from build123d import *

# Parameters (mm, degrees)
BOSS_EXTRUDE1_DEPTH     = 22.5
SKETCH2_R               = 7
CUT_EXTRUDE1_DEPTH      = 142.089510595
CUT_EXTRUDE2_DEPTH      = 150.198693024
CUT_EXTRUDE2_DEPTH_BACK = 150.198693024
SKETCH5_R               = 7
CHAMFER2_SIZE           = 1
FILLET2_R               = 1.5


with BuildPart() as part:
    # Sketch1 → Boss-Extrude1 (new, symmetric)
    with BuildSketch(Plane.XY):
        with BuildLine():
            Line((-74, -9), (-74, 9))
            Line((-74, 9), (-45, 9))
            Line((-45, 9), (-45, 127))
            Line((-45, 127), (-1, 127))
            Line((-1, 127), (-1, 100.983328701))
            ThreePointArc((-1, 100.983328701), (0, 41), (1, 100.983328701))
            Line((1, 100.983328701), (1, 127))
            Line((1, 127), (45, 127))
            Line((45, 127), (45, 9))
            Line((45, 9), (74, 9))
            Line((74, 9), (74, -9))
            Line((74, -9), (-74, -9))
        make_face()
    extrude(amount=BOSS_EXTRUDE1_DEPTH, both=True)

    # Sketch2 → Cut-Extrude1 (cut, through all)
    with BuildSketch(Plane(origin=(0, 9, 0), x_dir=(1, 0, 0), z_dir=(0, 1, 0))):
        with Locations(Location((60, 0, 0), (0, 0, 180))):
            Circle(SKETCH2_R)
        with Locations((-60, 0)):
            Circle(SKETCH2_R)
    extrude(amount=-CUT_EXTRUDE1_DEPTH, mode=Mode.SUBTRACT)

    # Sketch5 → Cut-Extrude2 (cut, two sides: drawn at the far end of the back side and taken through both)
    with BuildSketch(Plane(origin=(-1, 0, 0), x_dir=(0, 0, -1), z_dir=(1, 0, 0)).offset(-CUT_EXTRUDE2_DEPTH_BACK)):
        with Locations(Location((0.330734984, 113.991664351, 0), (0, 0, 90))):
            Circle(SKETCH5_R)
    extrude(amount=CUT_EXTRUDE2_DEPTH + CUT_EXTRUDE2_DEPTH_BACK, mode=Mode.SUBTRACT)

    # Chamfer2
    chamfer2_edges = [part.edges().sort_by_distance(p)[0] for p in [
        (0, 41, -22.5),
        (0, 41, 22.5),
        (67, 9, 0),
        (-67, 9, 0),
        (-45, 106.991664351, -0.330734984),
        (45, 106.991664351, -0.330734984),
    ]]
    chamfer(chamfer2_edges, length=CHAMFER2_SIZE)

    # Fillet2
    fillet2_edges = [part.edges().sort_by_distance(p)[0] for p in [
        (-59.5, 9, 22.5),
        (45, 68, -22.5),
        (59.5, 9, -22.5),
        (-74, 0, 22.5),
        (74, 0, -22.5),
        (-74, 0, -22.5),
        (-59.5, 9, -22.5),
        (-45, 68, -22.5),
        (74, 0, 22.5),
        (45, 127, 0),
        (74, 9, 0),
        (74, -9, 0),
        (-74, -9, 0),
        (-74, 9, 0),
        (-45, 127, 0),
        (59.5, 9, 22.5),
        (45, 68, 22.5),
        (-45, 68, 22.5),
    ]]
    fillet(fillet2_edges, radius=FILLET2_R)


solid = part.part
The model under review builds one solid part; all positions refer to its coordinate system, in mm. A direction names the side the tool comes from. Round coordinates to 2 decimals unless told otherwise and drop trailing zeros. Order: outer loops, then holes, each group sorted by start corner. A loop starts at its lowest first (then second) coordinate and runs counter-clockwise, first axis right, second up. Notation, with made-up numbers: (3.25, 69.25) -> (33.25, 69.25) arc R26 cw to (33.25, 99.25) -> close; hole circle Ø3 at (82, 15). An arc over 180 degrees is marked (long way). Write item = value, one per line. Start each with the question number.
Item 1: Mouldability with a two-part tool opening along X and no side actions: class faces 5 (the face through (-45, 66, 0)), 6 (the face through (17.1, 44.8, 22.5)), 7 (the face through (-1.31, 40.87, -21.66)), 8 (the face through (-53.323, -0.381, -2.103)) as released by +X, released by -X, zero draft, split by the parting line, or undercut.
Item 2: Consider section C-C on z = 18. Write out the cut boundary in (x, y).
Item 3: Clearance check with flat-ended pins moving along their axes: pin 1 Ø8 at (x, z) = (52, 4.5) entering from +Y; pin 2 Ø1.5 at (y, z) = (87, 6) entering from -X; pin 3 Ø13 at (y, z) = (112, 2) entering from +X. State where each tip first meets the part, or that it passes through.
Item 4: Consider section A-A on x = 60. Write out the cut boundary in (y, z).
Item 5: Consider section D-D on y = 0.5. Write out the cut boundary in (x, z).
Item 6: Consider section B-B on y = 71. Write out the cut boundary in (x, z), plus the area to 3 significant figures.
Item 7: For faces 1 (the face through (-1, 120, 5)), 2 (the face through (-74, 0, 0)), 3 (the face through (45, 68, 0)), 4 (the face through (-53, 9, 5)), list the 3-axis set-ups (+Z, -Z, +X, -X, +Y, -Y) from which the entire face can be reached by the end or side of a thin tool; tool diameter is ignored.
Item 8: For line 1 along Z through (x, y) = (60, 4.5); line 2 along Y through (x, z) = (-3, 5); line 3 along X through (y, z) = (106, 0), list the stretches that pass through material, from the lowest coordinate up.
Conclusion:
q1.face_5 = released by -X
q1.face_6 = zero draft
q1.face_7 = undercut
q1.face_8 = undercut
q2.outline = (-74, -7.5) arc R1.5 ccw to (-72.5, -9) -> (72.5, -9) arc R1.5 ccw to (74, -7.5) -> (74, 7.5) arc R1.5 ccw to (72.5, 9) -> (45, 9) -> (45, 125.5) arc R1.5 ccw to (43.5, 127) -> (1, 127) -> (1, 100.98) arc R30 cw (long way) to (-1, 100.98) -> (-1, 127) -> (-43.5, 127) arc R1.5 ccw to (-45, 125.5) -> (-45, 9) -> (-72.5, 9) arc R1.5 ccw to (-74, 7.5) -> close
q3.pin_1 = 9
q3.pin_2 = -45
q3.pin_3 = 45
q4.outline = (-9, -22.5) -> (7.5, -22.5) arc R1.5 ccw to (9, -21) -> (9, -8) -> (8, -7) -> (-9, -7) -> close; (-9, 7) -> (8, 7) -> (9, 8) -> (9, 21) arc R1.5 ccw to (7.5, 22.5) -> (-9, 22.5) -> close
q5.outline = (-74, -21) arc R1.5 ccw to (-72.5, -22.5) -> (72.5, -22.5) arc R1.5 ccw to (74, -21) -> (74, 21) arc R1.5 ccw to (72.5, 22.5) -> (-72.5, 22.5) arc R1.5 ccw to (-74, 21) -> close; hole circle Ø14 at (-60, 0); hole circle Ø14 at (60, 0)
q6.outline = (-45, -21) arc R1.5 ccw to (-43.5, -22.5) -> (-31, -22.5) -> (-30, -21.5) -> (-30, 21.5) -> (-31, 22.5) -> (-43.5, 22.5) arc R1.5 ccw to (-45, 21) -> close; (30, -21.5) -> (31, -22.5) -> (43.5, -22.5) arc R1.5 ccw to (45, -21) -> (45, 21) arc R1.5 ccw to (43.5, 22.5) -> (31, 22.5) -> (30, 21.5) -> close
q6.area = 1,350 mm2
q7.face_1 = +Z, -Z, +Y
q7.face_2 = +Z, -Z, -X, +Y, -Y
q7.face_3 = +Z, -Z, +X, +Y
q7.face_4 = +Z, -Z, -X, +Y
q8.line_1 = -22.5 to -7, 7 to 22.5
q8.line_2 = -9 to 41.15, 100.85 to 109.45, 118.53 to 127
q8.line_3 = -45 to -1, 1 to 45
